from build123d import *

# Parameters (mm, degrees)
F2_DEPTH      = 4
F5_DEPTH      = 49.55
F5_DEPTH_BACK = 53.25
F6_R          = 3.25
F6_R_2        = 1.75
F7_DEPTH      = 35.314708499
F8_DEPTH      = 5
F9_R          = 1.75
F9_W          = 23
F9_H          = 9.5
F10_DEPTH     = 4.001
F11_DEPTH     = 1
F12_T1_DEPTH  = 21.6004404508
F12_T3_DEPTH  = 86.8
F12_T5_DEPTH  = 21.6004404508
F12_T7_DEPTH  = 44.2278574488
F12_T9_DEPTH  = 35.0844914729
F12_T14_DEPTH = 15.9435862014
F12_T19_DEPTH = 15.9435862014
F12_T25_DEPTH = 98.9490097203
F12_S28_R     = 3.25
F12_T29_DEPTH = 51
F12_T32_DEPTH = 10.8002202254
F12_T39_DEPTH = 10.8002202254
F12_T43_DEPTH = 98.9490097203


# Not quite as in the source:
# - a fillet or chamfer that OpenCascade refuses, or shapes differently, is made with other operations: its cross-section is extruded or revolved along the edge and cut away or added


with BuildPart() as f2:
    # F0 (on Right) → F2 (new body, symmetric)
    with BuildSketch(Plane.YZ):
        Polygon((-8, 41.941125497), (-24.9705627485, 24.9705627485), (-41.941125497, 8), (-33.941125497, 0), (-4, 0), (-4, 37.941125497), align=None)
    extrude(amount=F2_DEPTH, both=True)


with BuildPart() as f3_1:
    # F3: copy of F2
    add(f2.part.moved(Location((-49.25, 0, 0))))


with BuildPart() as f2_1:
    # F4: moved
    add(f2.part.moved(Location((45.55, 0, 0))))


    add(f3_1.part)  # F5 merges F3_1
    # F0 (on Right) → F5 (join, two sides)
    with BuildSketch(Plane.YZ) as f5_sk:
        Polygon((0, 33.941125497), (-4, 37.941125497), (-4, 0), (0, 0), align=None)
    extrude(amount=F5_DEPTH)
    extrude(f5_sk.sketch, amount=-F5_DEPTH_BACK)

    # F6 (on line) → F7 (cut, through all)
    with BuildSketch(Plane(origin=(0, -24.9705627485, 24.9705627485), x_dir=(1, 0, 0), z_dir=(0, -0.7071067812, 0.7071067812))):
        with Locations((-49.25, 10.2)):
            Circle(F6_R)
        with Locations((-49.25, 10.2)):
            Circle(F6_R_2, mode=Mode.SUBTRACT)
        with Locations((-49.25, 10.2)):
            Circle(F6_R_2)
        with Locations((-49.25, -10.2)):
            Circle(F6_R)
        with Locations((-49.25, -10.2)):
            Circle(F6_R_2, mode=Mode.SUBTRACT)
        with Locations((-49.25, -10.2)):
            Circle(F6_R_2)
        with Locations((45.55, 19.5)):
            Circle(F6_R)
        with Locations((45.55, 19.5)):
            Circle(F6_R_2, mode=Mode.SUBTRACT)
        with Locations((45.55, 19.5)):
            Circle(F6_R_2)
        with Locations((45.55, -19.5)):
            Circle(F6_R)
        with Locations((45.55, -19.5)):
            Circle(F6_R_2, mode=Mode.SUBTRACT)
        with Locations((45.55, -19.5)):
            Circle(F6_R_2)
    extrude(amount=-F7_DEPTH, mode=Mode.SUBTRACT)

    # F6 (on line) → F8 (join)
    with BuildSketch(Plane(origin=(0, -24.9705627485, 24.9705627485), x_dir=(1, 0, 0), z_dir=(0, -0.7071067812, 0.7071067812))):
        with Locations((45.55, -19.5)):
            Circle(F6_R)
        with Locations((45.55, -19.5)):
            Circle(F6_R_2, mode=Mode.SUBTRACT)
        with Locations((45.55, 19.5)):
            Circle(F6_R)
        with Locations((45.55, 19.5)):
            Circle(F6_R_2, mode=Mode.SUBTRACT)
        with Locations((-49.25, 10.2)):
            Circle(F6_R)
        with Locations((-49.25, 10.2)):
            Circle(F6_R_2, mode=Mode.SUBTRACT)
        with Locations((-49.25, -10.2)):
            Circle(F6_R)
        with Locations((-49.25, -10.2)):
            Circle(F6_R_2, mode=Mode.SUBTRACT)
    extrude(amount=-F8_DEPTH)

    # F9 (on face) → F10 (cut, through all)
    with BuildSketch(Plane.XZ.offset(4)):
        with Locations((-35, 15)):
            Circle(F9_R)
        with Locations((35, 15)):
            Circle(F9_R)
        with Locations((23.75, 24.75)):
            Rectangle(F9_W, F9_H)
    extrude(amount=-F10_DEPTH, mode=Mode.SUBTRACT)

    # F9 (on face) → F11 (cut)
    with BuildSketch(Plane.XZ.offset(4)):
        Polygon((-32.15, 13.3545517328), (-32.15, 16.6454482672), (-35, 18.2908965344), (-37.85, 16.6454482672), (-37.85, 13.3545517328), (-35, 11.7091034656), align=None)
        with Locations((-35, 15)):
            Circle(F9_R, mode=Mode.SUBTRACT)
        Polygon((37.85, 13.3545517328), (37.85, 16.6454482672), (35, 18.2908965344), (32.15, 16.6454482672), (32.15, 13.3545517328), (35, 11.7091034656), align=None)
        with Locations((35, 15)):
            Circle(F9_R, mode=Mode.SUBTRACT)
    extrude(amount=-F11_DEPTH, mode=Mode.SUBTRACT)

    # F12: chamfer of 2 on 13 edges, made by hand

    # F12_s2 → F12_t1 (cut)
    with BuildSketch(Plane(origin=(0, -28.6074717082, 28.6074717082), x_dir=(1, 0, 0), z_dir=(0, 0.7071067812, -0.7071067812))):
        Polygon((47.55, -24), (49.55, -22), (49.55, -24), align=None)
        Polygon((-53.25, 22), (-51.25, 24), (-53.25, 24), align=None)
        Polygon((-45.25, 22), (-47.25, 24), (-45.25, 24), align=None)
        Polygon((41.55, 22), (43.55, 24), (41.55, 24), align=None)
        Polygon((49.55, 22), (47.55, 24), (49.55, 24), align=None)
    extrude(amount=F12_T1_DEPTH, mode=Mode.SUBTRACT)

    # F12_s4 → F12_t3 (cut)
    with BuildSketch(Plane.YZ.offset(-45.25)):
        Polygon((-0.5857864376, 34.5269119346), (-4, 33.1126983722), (-4, 37.941125497), align=None)
    extrude(amount=F12_T3_DEPTH, mode=Mode.SUBTRACT)

    # F12_s6 → F12_t5 (cut)
    with BuildSketch(Plane(origin=(0, -13.3336537888, 13.3336537888), x_dir=(1, 0, 0), z_dir=(0, -0.7071067812, 0.7071067812))):
        Polygon((-51.25, 24), (-53.25, 22), (-53.25, 24), align=None)
    extrude(amount=F12_T5_DEPTH, mode=Mode.SUBTRACT)

    # F12_s8 → F12_t7 (cut)
    with BuildSketch(Plane.XZ.offset(-5.1433659759)):
        Polygon((-53.25, 2), (-51.25, 0), (-53.25, 0), align=None)
        Polygon((49.55, 2), (47.55, 0), (49.55, 0), align=None)
    extrude(amount=F12_T7_DEPTH, mode=Mode.SUBTRACT)

    # F12_s10 → F12_t9 (cut)
    with BuildSketch(Plane.XZ.offset(4)):
        Polygon((-45.25, 2), (-47.25, 0), (-45.25, 0), align=None)
        Polygon((41.55, 2), (43.55, 0), (41.55, 0), align=None)
    extrude(amount=F12_T9_DEPTH, mode=Mode.SUBTRACT)


with BuildPart() as f12_tool12:
    # F12_s13 → F12_t14 (new body)
    with BuildSketch(Plane(origin=(0, -17.3336537888, 17.3336537888), x_dir=(1, 0, 0), z_dir=(0, -0.7071067812, 0.7071067812))):
        Polygon((-47.25, 24), (-45.25, 22), (-45.25, 24), align=None)
    extrude(amount=F12_T14_DEPTH)

    split(bisect_by=Plane.XZ.offset(4), keep=Keep.TOP)


with BuildPart() as f2_2:
    add(f2_1.part)

    # F12_t11: cut F12_tool12
    add(f12_tool12.part, mode=Mode.SUBTRACT)


with BuildPart() as f12_tool17:
    # F12_s18 → F12_t19 (new body)
    with BuildSketch(Plane(origin=(0, -17.3336537888, 17.3336537888), x_dir=(1, 0, 0), z_dir=(0, -0.7071067812, 0.7071067812))):
        Polygon((43.55, 24), (41.55, 22), (41.55, 24), align=None)
    extrude(amount=F12_T19_DEPTH)

    split(bisect_by=Plane.XZ.offset(4), keep=Keep.TOP)


with BuildPart() as f2_3:
    add(f2_2.part)

    # F12_t16: cut F12_tool17
    add(f12_tool17.part, mode=Mode.SUBTRACT)


with BuildPart() as f12_tool23:
    # F12_s24 → F12_t25 (new body)
    with BuildSketch(Plane.YZ.offset(53.6990097203)):
        Polygon((-0.5857864376, 34.5269119346), (-4, 33.1126983722), (-4, 37.941125497), align=None)
    extrude(amount=-F12_T25_DEPTH)

    split(bisect_by=Plane.YZ.offset(41.55), keep=Keep.TOP)

    split(bisect_by=Plane.YZ.offset(49.55), keep=Keep.BOTTOM)

    # F12_s28 → F12_t29 (cut, symmetric)
    with BuildSketch(Plane(origin=(0, -18.8797510577, 18.8797510577), x_dir=(1, 0, 0), z_dir=(0, -0.7071067812, 0.7071067812))):
        with Locations((45.55, 19.5)):
            Circle(F12_S28_R)
    extrude(amount=F12_T29_DEPTH, both=True, mode=Mode.SUBTRACT)


with BuildPart() as f12_tool30:
    # F12_s31 → F12_t32 (new body)
    with BuildSketch(Plane(origin=(0, -17.3336537888, 17.3336537888), x_dir=(1, 0, 0), z_dir=(0, -0.7071067812, 0.7071067812))):
        Polygon((43.55, 24), (41.55, 22), (41.55, 24), align=None)
    extrude(amount=F12_T32_DEPTH)

    split(bisect_by=Plane.XZ.offset(4), keep=Keep.BOTTOM)


with BuildPart() as f12_tool23_1:
    add(f12_tool23.part)

    # F12_t34: intersect F12_tool30
    add(f12_tool30.part, mode=Mode.INTERSECT)


with BuildPart() as f2_4:
    add(f2_3.part)

    # F12_t21: cut F12_tool23
    add(f12_tool23_1.part, mode=Mode.SUBTRACT)


with BuildPart() as f12_tool37:
    # F12_s38 → F12_t39 (new body)
    with BuildSketch(Plane(origin=(0, -17.3336537888, 17.3336537888), x_dir=(1, 0, 0), z_dir=(0, -0.7071067812, 0.7071067812))):
        Polygon((-47.25, 24), (-45.25, 22), (-45.25, 24), align=None)
    extrude(amount=F12_T39_DEPTH)

    split(bisect_by=Plane.XZ.offset(4), keep=Keep.BOTTOM)


with BuildPart() as f12_tool41:
    # F12_s42 → F12_t43 (new body)
    with BuildSketch(Plane.YZ.offset(41.55)):
        Polygon((-0.5857864376, 34.5269119346), (-4, 33.1126983722), (-4, 37.941125497), align=None)
    extrude(amount=-F12_T43_DEPTH)

    split(bisect_by=Plane.YZ.offset(-45.25), keep=Keep.BOTTOM)

    split(bisect_by=Plane.YZ.offset(-53.25), keep=Keep.TOP)


with BuildPart() as f12_tool37_1:
    add(f12_tool37.part)

    # F12_t46: intersect F12_tool41
    add(f12_tool41.part, mode=Mode.INTERSECT)


with BuildPart() as f2_5:
    add(f2_4.part)

    # F12_t35: cut F12_tool37
    add(f12_tool37_1.part, mode=Mode.SUBTRACT)


solid = f2_5.part
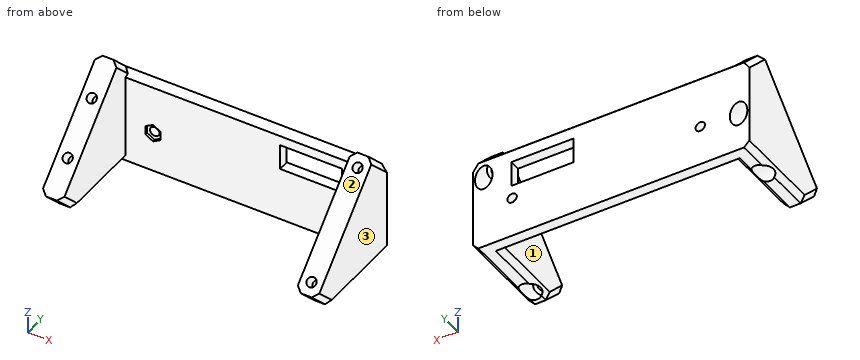
Model file for the job. Use its own axes, mm. Face numbers are marked on the shaded views. Give positions to 0.01 mm unless a question says otherwise; leave off trailing zeros. Answer as CSV lines item,"result".
1. Pin check, flat tips, straight feed: pin 1 (4 mm diameter, centred on x = 13, z = 29, fed in from -Y); pin 2 (1 mm diameter, centred on x = 30.5, z = 27.5, fed in from +Y). Stop position of each tip, or through.
Responses:
pin 1,"stops at y = -4"
pin 2,"passes through"
2. Two-plate mould, pull along X, no slides. Class the marked faces 1, 2 and 3: +X half, -X half, draft (parallel to the pull), parting line (faces both ways), or undercut.
Responses:
face 1,"undercut"
face 2,"draft"
face 3,"+X half"
3. Band-saw the part on A-A (z = 22). Count the separate pieces of the cut face and the enclosed holes in it, and give its area (3 significant figures).
Responses:
separate pieces,"2"
enclosed holes,"1"
area,"655 mm2"
4. Drill centre lines: L1, parallel to Z at x = 35, y = -1; L2, parallel to X at y = -6.5, z = 3; L3, parallel to Y at x = -32.5, z = 11. Where is each one in solid material? Low to high. Write a range as [from, to].
Responses:
L1,"z = [0, 13.25], [16.75, 20], [29.5, 34.36]"
L2,"x = [-53.25, -45.25], [41.55, 49.55]"
L3,"y = [-4, 0]"
